Verification items for the finished model (mm, model axes). Face numbers are marked on the shaded views. A direction names the side the tool comes from. Round coordinates to 2 decimals unless told otherwise and drop trailing zeros. Write each loop counter-clockwise with the first axis right and the second up, starting at its lowest first coordinate (ties: lowest second). Pieces come first, ordered by that corner, then holes.
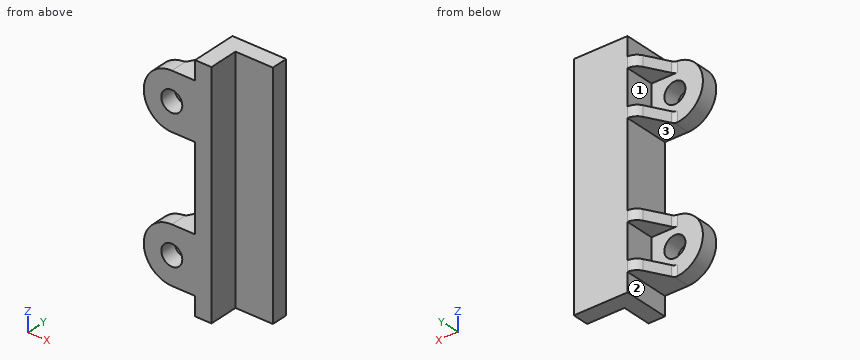
from build123d import *

# Parameters (mm, degrees)
SALIENTE_EXTRUIR1_DEPTH  = 25
CROQUIS2_R               = 2.25
SALIENTE_EXTRUIR2_DEPTH  = 3.5
SALIENTE_EXTRUIR3_DEPTH  = 2.25
REDONDEO3_R              = 1
REDONDEO5_R              = 2.5
REDONDEO3_OF_SIMETR_A1_R = 1
REDONDEO5_OF_SIMETR_A1_R = 2.5
REDONDEO3_OF_SIMETR_A4_R = 1
REDONDEO5_OF_SIMETR_A4_R = 2.5
SALIENTE_EXTRUIR4_DEPTH  = 2.25
REDONDEO6_R              = 2.5
REDONDEO7_R              = 1


with BuildPart() as part:
    # Croquis1 → Saliente-Extruir1 (new, symmetric)
    with BuildSketch(Plane.XY):
        Polygon((0, 0), (0, 9.8), (11.5, 9.8), (11.5, 6.3), (3.5, 6.3), (3.5, 0), align=None)
    extrude(amount=SALIENTE_EXTRUIR1_DEPTH, both=True)

    # Croquis2 → Saliente-Extruir2 (add)
    with BuildSketch(Plane(origin=(0, 0, 0), x_dir=(1, 0, 0), z_dir=(0, 1, 0))):
        with BuildLine():
            Line((0, 9), (-5, 9))
            ThreePointArc((-5, 9), (-11, 15), (-5, 21))
            Line((-5, 21), (0, 21))
            Line((0, 21), (0, 9))
        make_face()
        with Locations(Location((-5, 15, 0), (0, 0, 270))):
            Circle(CROQUIS2_R, mode=Mode.SUBTRACT)
    saliente_extruir2 = extrude(amount=SALIENTE_EXTRUIR2_DEPTH)

    # Croquis3 → Saliente-Extruir3 (add)
    with BuildSketch(Plane.XY.offset(-9)):
        Polygon((0, 9.8), (0, 3.5), (-5, 3.5), (-1.5, 9.8), align=None)
    saliente_extruir3 = extrude(amount=-SALIENTE_EXTRUIR3_DEPTH)

    # Redondeo3
    redondeo3_edges = [part.edges().sort_by_distance(p)[0] for p in [
        (-5, 3.5, -10.125),
    ]]
    fillet(redondeo3_edges, radius=REDONDEO3_R)

    # Redondeo5
    redondeo5_edges = [part.edges().sort_by_distance(p)[0] for p in [
        (-1.5, 9.8, -10.125),
    ]]
    fillet(redondeo5_edges, radius=REDONDEO5_R)

    # Simetría1: Saliente-Extruir3 across plane
    add(saliente_extruir3.mirror(Plane(origin=(0, 0, -15), x_dir=(1, 0, 0), z_dir=(0, 0, -1))))

    # Redondeo3 of Simetría1
    redondeo3_of_simetr_a1_edges = [part.edges().sort_by_distance(p)[0] for p in [
        (-5, 3.5, -19.875),
    ]]
    fillet(redondeo3_of_simetr_a1_edges, radius=REDONDEO3_OF_SIMETR_A1_R)

    # Redondeo5 of Simetría1
    redondeo5_of_simetr_a1_edges = [part.edges().sort_by_distance(p)[0] for p in [
        (-1.5, 9.8, -19.875),
    ]]
    fillet(redondeo5_of_simetr_a1_edges, radius=REDONDEO5_OF_SIMETR_A1_R)

    # Simetría4: Saliente-Extruir2, Saliente-Extruir3 across plane
    add(saliente_extruir2.mirror(Plane.XY))
    add(saliente_extruir3.mirror(Plane.XY))

    # Redondeo3 of Simetría4
    redondeo3_of_simetr_a4_edges = [part.edges().sort_by_distance(p)[0] for p in [
        (-5, 3.5, 10.125),
    ]]
    fillet(redondeo3_of_simetr_a4_edges, radius=REDONDEO3_OF_SIMETR_A4_R)

    # Redondeo5 of Simetría4
    redondeo5_of_simetr_a4_edges = [part.edges().sort_by_distance(p)[0] for p in [
        (-1.5, 9.8, 10.125),
    ]]
    fillet(redondeo5_of_simetr_a4_edges, radius=REDONDEO5_OF_SIMETR_A4_R)

    # Croquis4 → Saliente-Extruir4 (add)
    with BuildSketch(Plane.XY.offset(21)):
        Polygon((0, 3.5), (-5, 3.5), (-1.5, 9.8), (0, 9.8), align=None)
    extrude(amount=-SALIENTE_EXTRUIR4_DEPTH)

    # Redondeo6
    redondeo6_edges = [part.edges().sort_by_distance(p)[0] for p in [
        (-1.5, 9.8, 19.875),
    ]]
    fillet(redondeo6_edges, radius=REDONDEO6_R)

    # Redondeo7
    redondeo7_edges = [part.edges().sort_by_distance(p)[0] for p in [
        (-5, 3.5, 19.875),
    ]]
    fillet(redondeo7_edges, radius=REDONDEO7_R)


solid = part.part
Q1. Depth check by flat-ended pin: P1, Ø4, axis at x = -5, z = 15, coming from the -Y side; P2, Ø3.5, axis at x = -3.5, z = -14.5, coming from the +Y side; P3, Ø1.5, axis at x = -5, y = 4.5, coming from the -Z side; P4, Ø1.5, axis at y = 3.5, z = 8, coming from the +X side. Enter the tip coordinate at first touch or a pass-through.
Recorded:
P1: passes through
P2: stops at y = 3.5
P3: stops at z = -21
P4: stops at x = 3.5
Q2. Sectioned sample at B-B (y = 2.25). Enter the section's corners in (x, z), plus the area to 3 significant figures.
Recorded:
outline: (-5, -21) - (0, -21) - (0, -25) - (3.5, -25) - (3.5, 25) - (0, 25) - (0, 21) - (-5, 21) arc R6 ccw to (-5, 9) - (0, 9) - (0, -9) - (-5, -9) arc R6 ccw to start; hole circle Ø4.5 at (-5, -15); hole circle Ø4.5 at (-5, 15)
area: 376 mm2
Q3. Sectioned sample at A-A (z = 15). Enter the section's corners in (x, y).
Recorded:
outline: (-11, 0) - (-7.25, 0) - (-7.25, 3.5) - (-11, 3.5) - close; (-2.75, 0) - (3.5, 0) - (3.5, 6.3) - (11.5, 6.3) - (11.5, 9.8) - (0, 9.8) - (0, 3.5) - (-2.75, 3.5) - close
Q4. Tool access check on the marked faces 1, 2 and 3. Record the directions out of +Z, -Z, +X, -X, +Y, -Y that give a thin tool (end or side, any length) a straight path to the whole face; none if there is none.
Recorded:
face 1: -X, +Y
face 2: -Z, -X, +Y, -Y
face 3: -X, +Y, -Y
Q5. Material ranges on line 1 along Z through (x, y) = (-2, 7.75); line 2 along X through (y, z) = (1.7, 15); line 3 along Y through (x, z) = (5, -10), recorded low to high.
Recorded:
line 1: z = -21 to -18.75, -11.25 to -9, 9 to 11.25, 18.75 to 21
line 2: x = -11 to -7.25, -2.75 to 3.5
line 3: y = 6.3 to 9.8
Q6. Sectioned sample at D-D (x = 7.25). Enter the section's corners in (y, z).
Recorded:
outline: (6.3, -25) - (9.8, -25) - (9.8, 25) - (6.3, 25) - close
Q7. Sectioned sample at C-C (z = -16.5). Enter the section's corners in (x, y), plus the area to 3 significant figures.
Recorded:
outline: (-10.81, 0) - (-6.68, 0) - (-6.68, 3.5) - (-10.81, 3.5) - close; (-3.32, 0) - (3.5, 0) - (3.5, 6.3) - (11.5, 6.3) - (11.5, 9.8) - (0, 9.8) - (0, 3.5) - (-3.32, 3.5) - close
area: 88.4 mm2
